from build123d import *

# Parameters (mm, degrees)
SKETCH1_W           = 25
SKETCH1_H           = 15
BOSS_EXTRUDE1_DEPTH = 0.3
SKETCH2_W           = 3
SKETCH2_H           = 15
BOSS_EXTRUDE2_DEPTH = 3
SKETCH2_5_R         = 1.5
CUT_EXTRUDE1_DEPTH  = 3


with BuildPart() as part:
    # Sketch1 → Boss-Extrude1 (new body)
    with BuildSketch(Plane(origin=(0, 0, 0), x_dir=(1, 0, 0), z_dir=(0, 1, 0))):
        with Locations((12.5, 7.5)):
            Rectangle(SKETCH1_W, SKETCH1_H)
    extrude(amount=BOSS_EXTRUDE1_DEPTH)

    # Sketch2 → Boss-Extrude2 (add)
    with BuildSketch(Plane(origin=(0, 0.3, 0), x_dir=(1, 0, 0), z_dir=(0, 1, 0))):
        with Locations((12.5, 7.5)):
            Rectangle(SKETCH2_W, SKETCH2_H)
    extrude(amount=BOSS_EXTRUDE2_DEPTH)

    # Sketch2_5 → Cut-Extrude1 (cut)
    with BuildSketch(Plane(origin=(0, 0.3, 0), x_dir=(1, 0, 0), z_dir=(0, 1, 0))):
        with Locations(Location((6, 7.5, 0), (0, 0, 270))):
            Circle(SKETCH2_5_R)
    extrude(amount=-CUT_EXTRUDE1_DEPTH, mode=Mode.SUBTRACT)


solid = part.part
Could you check a few things on this model? Use its own coordinates, in mm. A direction names the side the tool comes from. Coordinates: 2 decimals unless noted, no trailing zeros. Order: outer loops, then holes, each group sorted by start corner. A loop starts at its lowest first (then second) coordinate and runs counter-clockwise, first axis right, second up. Notation, with made-up numbers: (55.25, 3) -> (61.25, 3) arc R20 cw to (61.25, 33) -> close; hole circle Ø1 at (-23, -35). An arc over 180 degrees is marked (long way). One line per item, written item: value. Start each with the question number.
1) Imagine slicing it at D-D on y = 1.95. List the corners of the cut face in (x, z) for me, plus the area to 3 significant figures.
2) I'm going to push flat-ended pins straight in: pin 1 (3.5 mm diameter, centred on x = 19, z = -9, fed in from +Y); pin 2 (0.9 mm diameter, centred on y = 1.5, z = -8.5, fed in from -X). Where does each tip first touch, or does it pass through?
3) Which directions (+Z, -Z, +X, -X, +Y, -Y) give clear straight access to the entire face, cutting with the end or side of a thin tool? Please do faces 1 (the flat face through (19, 0.3, -8)), 2 (the flat face through (11, 2, -7)), 3 (the flat face through (12, 1, -15)).
4) Imagine slicing it at B-B on x = 6. List the corners of the cut face in (y, z) for me.
5) We'd pull the mould along X, two halves only. Please class faces 4 (the flat face through (12, 3.3, -8)), 5 (the flat face through (14, 2, -7)), 6 (the cylindrical face through (5.09, 0.15, -8.69)): +X half, -X half, draft (parallel to the pull), parting line (faces both ways), or undercut.
6) Imagine slicing it at C-C on z = -0.75. List the corners of the cut face in (x, y) for me.
7) If I drill on L1, parallel to X at y = 0.15, z = -7.5; L2, parallel to Y at x = 5, z = -1; L3, parallel to X at y = 2.1, z = -0.25, over which ranges is the centre line in solid material (lowest first)? Write a range as [from, to].
8) Imagine slicing it at A-A on z = -7.5. List the corners of the cut face in (x, y) for me, plus the area to 3 significant figures.
Answer list:
1. outline: (11, -15) -> (14, -15) -> (14, 0) -> (11, 0) -> close
1. area: 45.0 mm2
2. pin 1: stops at y = 0.3
2. pin 2: stops at x = 11
3. face 1: +Z, -Z, +X, +Y
3. face 2: +Z, -Z, -X, +Y
3. face 3: -Z, +X, -X, +Y, -Y
4. outline: (0, -15) -> (0.3, -15) -> (0.3, -9) -> (0, -9) -> close; (0, -6) -> (0.3, -6) -> (0.3, 0) -> (0, 0) -> close
5. face 4: draft
5. face 5: +X half
5. face 6: undercut
6. outline: (0, 0) -> (25, 0) -> (25, 0.3) -> (14, 0.3) -> (14, 3.3) -> (11, 3.3) -> (11, 0.3) -> (0, 0.3) -> close
7. L1: x = [0, 4.5], [7.5, 25]
7. L2: y = [0, 0.3]
7. L3: x = [11, 14]
8. outline: (0, 0) -> (4.5, 0) -> (4.5, 0.3) -> (0, 0.3) -> close; (7.5, 0) -> (25, 0) -> (25, 0.3) -> (14, 0.3) -> (14, 3.3) -> (11, 3.3) -> (11, 0.3) -> (7.5, 0.3) -> close
8. area: 15.6 mm2
